Source: CAD feature listing. Evaluate the final solid. Frame: model axes, mm. Face numbers are marked on the shaded views. A direction names the side the tool comes from. Round coordinates to 2 decimals unless told otherwise and drop trailing zeros. Write each loop counter-clockwise with the first axis right and the second up, starting at its lowest first coordinate (ties: lowest second). Pieces come first, ordered by that corner, then holes. Notation, with made-up numbers: (40, 15) - (98, 15) arc R17 cw to (98, 37) - close; hole circle Ø7 at (-10.75, -1.5). An arc over 180 degrees is marked (long way). Write item = value, one per line. Start each with the question number.
```python
from build123d import *

# Parameters (mm, degrees)
ESQUISSE1_R             = 1.5
BOSS_EXTRU_1_DEPTH      = 3
ESQUISSE2_W             = 9
ESQUISSE2_H             = 3
BOSS_EXTRU_2_DEPTH      = 12
ESQUISSE3_R             = 2
ENL_V_MAT_EXTRU_1_DEPTH = 25.211832251
CONG_1_R                = 3


with BuildPart() as part:
    # Esquisse1 → Boss.-Extru.1 (new body)
    with BuildSketch(Plane.XY):
        with BuildLine():
            Line((-18.115, 7.3), (-18.115, 0))
            Line((-18.115, 0), (18.115, 0))
            Line((18.115, 0), (18.115, 7.3))
            ThreePointArc((18.115, 7.3), (14.615, 8.749747468), (11.115, 7.3))
            Line((11.115, 7.3), (11.115, 3))
            Line((11.115, 3), (-11.115, 3))
            Line((-11.115, 3), (-11.115, 7.3))
            ThreePointArc((-11.115, 7.3), (-14.615, 8.749747468), (-18.115, 7.3))
        make_face()
        with Locations((-14.615, 3.8)):
            Circle(ESQUISSE1_R, mode=Mode.SUBTRACT)
        with Locations((14.615, 3.8)):
            Circle(ESQUISSE1_R, mode=Mode.SUBTRACT)
    extrude(amount=BOSS_EXTRU_1_DEPTH)

    # Esquisse2 → Boss.-Extru.2 (add)
    with BuildSketch(Plane.XY.offset(3)):
        with Locations((0, 1.5)):
            Rectangle(ESQUISSE2_W, ESQUISSE2_H)
    extrude(amount=BOSS_EXTRU_2_DEPTH)

    # Esquisse3 → Enlèv. mat.-Extru.1 (cut, through all)
    with BuildSketch(Plane(origin=(0, 3, 0), x_dir=(1, 0, 0), z_dir=(0, 1, 0))):
        with Locations(Location((0, -9, 0), (0, 0, 270))):
            Circle(ESQUISSE3_R)
    extrude(amount=-ENL_V_MAT_EXTRU_1_DEPTH, mode=Mode.SUBTRACT)

    # Congé1
    cong_1_edges = [part.edges().sort_by_distance(p)[0] for p in [
        (-11.115, 3, 1.5),
        (11.115, 3, 1.5),
        (-4.5, 1.5, 3),
        (4.5, 1.5, 3),
        (-4.5, 1.5, 15),
        (4.5, 1.5, 15),
    ]]
    fillet(cong_1_edges, radius=CONG_1_R)


solid = part.part
```
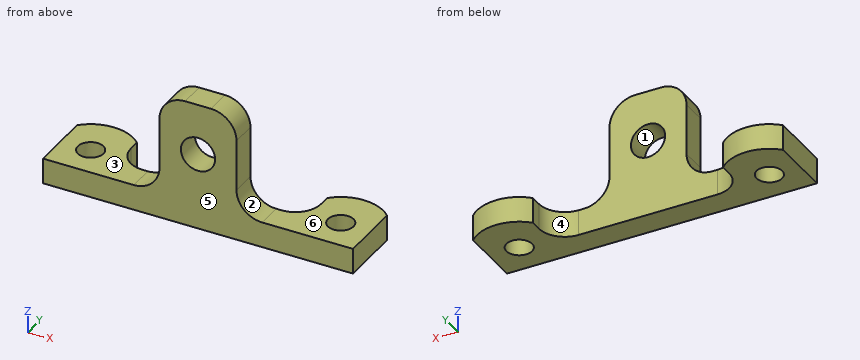
(1) Pull-direction query (X, two-part tool) for the marked faces 1, 2 and 3; classes: +X half, -X half, draft (parallel to the pull), parting line (faces both ways), or undercut.
(2) Section B-B (z = 10.5). Return the cut outline in (x, y), plus the area to 3 significant figures.
(3) Ray query, L1, parallel to X at y = 0.7, z = 9; L2, parallel to X at y = 2.5, z = 8.5; L3, parallel to Y at x = 1, z = 4.75. Return the intervals inside material, ascending. Write a range as from..to.
(4) Contact query for flat-ended pins moving along their axis: P1, Ø1.5, axis at x = -1, z = 11.5, coming from the +Y side; P2, Ø2, axis at y = 1.5, z = 7, coming from the +X side; P3, Ø1, axis at x = 1, y = 5, coming from the -Z side; P4, Ø4, axis at x = 14.615, y = 3.8, coming from the +Z side. Output: stop coordinate, or through.
(5) Section A-A (x = 0). Return the cut outline in (y, z), plus the area to 3 significant figures.
(6) Section D-D (y = 3.8). Return the cut outline in (x, z) (3 decimals), plus the area to 3 significant figures.
(7) Section C-C (y = 1.75). Return the cut outline in (x, z) (3 decimals).
(8) Reachability of the marked faces 4, 5 and 6 from +Z, -Z, +X, -X, +Y, -Y: full face, straight path, thin tool, end or side. Return the list, or none.
Solution:
q1.face_1 = undercut
q1.face_2 = +X half
q1.face_3 = draft
q2.outline = (-4.5, 0) - (-1.32, 0) - (-1.32, 3) - (-4.5, 3) - close; (1.32, 0) - (4.5, 0) - (4.5, 3) - (1.32, 3) - close
q2.area = 19.1 mm^2
q3.L1 = -4.5..-2, 2..4.5
q3.L2 = -4.5..-1.94, 1.94..4.5
q3.L3 = 0..3
q4.P1 = 3
q4.P2 = 4.5
q4.P3 = through
q4.P4 = 3
q5.outline = (0, 0) - (3, 0) - (3, 7) - (0, 7) - close; (0, 11) - (3, 11) - (3, 15) - (0, 15) - close
q5.area = 33.0 mm^2
q6.outline = (-18.115, 0) - (-16.115, 0) - (-16.115, 3) - (-18.115, 3) - close; (-13.115, 0) - (-10.155, 0) - (-10.155, 3) - (-13.115, 3) - close; (10.155, 0) - (13.115, 0) - (13.115, 3) - (10.155, 3) - close; (16.115, 0) - (18.115, 0) - (18.115, 3) - (16.115, 3) - close
q6.area = 29.8 mm^2
q7.outline = (-18.115, 0) - (18.115, 0) - (18.115, 3) - (7.5, 3) arc R3 cw to (4.5, 6) - (4.5, 12) arc R3 ccw to (1.5, 15) - (-1.5, 15) arc R3 ccw to (-4.5, 12) - (-4.5, 6) arc R3 cw to (-7.5, 3) - (-18.115, 3) - close; hole circle Ø4 at (0, 9)
q8.face_4 = +Z, -Z, +Y
q8.face_5 = +Z, -Z, +X, -X, -Y
q8.face_6 = +Z, +X, +Y, -Y
